from build123d import *

# Parameters (mm, degrees)
SZKIC1_R                    = 8.5
SZKIC1_R_2                  = 1.5
DODANIE_WYCI_GNI_CIE1_DEPTH = 5
SFAZOWANIE2_SIZE            = 0.5


with BuildPart() as part:
    # Szkic1 → Dodanie-wyciągnięcie1 (new body)
    with BuildSketch(Plane.XY):
        Polygon((-14, -12), (-14, 8), (-3.5, 20), (-3.5, 40), (23.5, 40), (48, 8), (48, -12), align=None)
        Circle(SZKIC1_R, mode=Mode.SUBTRACT)
        with Locations((34, 0)):
            Circle(SZKIC1_R, mode=Mode.SUBTRACT)
        with Locations((11.5, 23)):
            Circle(SZKIC1_R, mode=Mode.SUBTRACT)
        with Locations((12.5, 37)):
            Circle(SZKIC1_R_2, mode=Mode.SUBTRACT)
        with Locations((17, 0)):
            Circle(SZKIC1_R_2, mode=Mode.SUBTRACT)
    extrude(amount=DODANIE_WYCI_GNI_CIE1_DEPTH)

    # Sfazowanie2
    sfazowanie2_edges = [part.edges().sort_by_distance(p)[0] for p in [
        (-8.5, 0, 5),
        (25.5, 0, 5),
        (3, 23, 5),
    ]]
    chamfer(sfazowanie2_edges, length=SFAZOWANIE2_SIZE)


solid = part.part
The listing builds one solid part. Answer for the finished solid, in the listing's coordinates (mm). A direction names the side the tool comes from. Coordinates: 2 decimals unless noted, no trailing zeros. Order: outer loops, then holes, each group sorted by start corner. A loop starts at its lowest first (then second) coordinate and runs counter-clockwise, first axis right, second up.
Q1. Given P1, Ø15.5, axis at x = 11.5, y = 23, coming from the +Z side; P2, Ø1.5, axis at x = 36.5, z = 3.5, coming from the +Y side; P3, Ø1.5, axis at y = 23, z = 3.5, coming from the -X side, each flat-ended and moving along its own axis, determine where each tip first touches the part or whether it passes through.
Q2. A cutting plane is placed at A-A, the plane x = 0. Write down the section's boundary in (y, z).
Q3. Which of the six approach directions +Z, -Z, +X, -X, +Y, -Y give full straight-line access (tool end or side, diameter ignored) to faces 4 (the face through (17, 9, 5)), 5 (the face through (-3.5, 30, 2))?
Q4. A cutting plane is placed at D-D, the plane y = 0. Write down the section's boundary in (x, z), and give its area (4 significant figures).
Q5. A cutting plane is placed at C-C, the plane z = 0.65. Write down the section's boundary in (x, y), and give its area (3 significant figures).
Q6. Consider line 1 (Y direction, x = 0, z = 2.25); line 2 (Y direction, x = 17, z = 3.75); line 3 (X direction, y = 1, z = 1.75). Determine where each line is inside the solid, lowest interval first.
Q7. For a pull along X with two mould halves and no side action, classify faces 1 (the face through (-8.82, 13.92, 2.46)), 2 (the face through (15.5, 0.07, 2.46)), 3 (the face through (17, 14, 0)) as pulls with the +X half, pulls with the -X half, needs draft (parallel to the pull), parting line crosses it, or undercut.
Q8. A cutting plane is placed at B-B, the plane y = 23. Write down the section's boundary in (x, z), and give its area (3 significant figures).
Answers follow:
1. P1: passes through
1. P2: stops at y = 24
1. P3: stops at x = -3.5
2. outline: (-12, 0) - (-8.5, 0) - (-8.5, 4.5) - (-9, 5) - (-12, 5) - close; (8.5, 0) - (40, 0) - (40, 5) - (9, 5) - (8.5, 4.5) - close
3. face 4: +Z, +X, -X, +Y, -Y
3. face 5: +Z, -Z, -X, +Y
4. outline: (-14, 0) - (-8.5, 0) - (-8.5, 4.5) - (-9, 5) - (-14, 5) - close; (8.5, 0) - (15.5, 0) - (15.5, 5) - (9, 5) - (8.5, 4.5) - close; (18.5, 0) - (25.5, 0) - (25.5, 4.5) - (25, 5) - (18.5, 5) - close; (42.5, 0) - (48, 0) - (48, 5) - (43, 5) - (42.5, 4.5) - close
4. area: 124.5 mm2
5. outline: (-14, -12) - (48, -12) - (48, 8) - (23.5, 40) - (-3.5, 40) - (-3.5, 20) - (-14, 8) - close; hole circle Ø17 at (0, 0); hole circle Ø17 at (11.5, 23); hole circle Ø3 at (12.5, 37); hole circle Ø3 at (17, 0); hole circle Ø17 at (34, 0)
5. area: 1,860 mm2
6. line 1: y = -12 to -8.5, 8.5 to 40
6. line 2: y = -12 to -1.5, 1.5 to 16.52, 29.48 to 40
6. line 3: x = -14 to -8.44, 8.44 to 15.88, 18.12 to 25.56, 42.44 to 48
7. face 1: pulls with the -X half
7. face 2: undercut
7. face 3: needs draft
8. outline: (-3.5, 0) - (3, 0) - (3, 4.5) - (2.5, 5) - (-3.5, 5) - close; (20, 0) - (36.52, 0) - (36.52, 5) - (20.5, 5) - (20, 4.5) - close
8. area: 115 mm2
